from build123d import *

# Parameters (mm, degrees)
F1_DEPTH = 8
F3_DEPTH = 3
F4_R     = 1.5


with BuildPart() as f1:
    # F0 (on Right) → F1 (new body)
    with BuildSketch(Plane.YZ):
        Polygon((0, 14.684157), (-17.555564, 0), (17.444436, 0), align=None)
    extrude(amount=F1_DEPTH)

    # F2 (on face) → F3 (cut)
    with BuildSketch(Plane.YZ.offset(8)):
        Polygon((-0.5, 11.925979), (-12.543837, 1.82), (-7.876665, 1.82), (-4.89646, 4.320689), (-2.798133, 1.82), (-0.5, 3.748363), (-2.598327, 6.249052), (-0.5, 8.009757), align=None)
        Polygon((2.5, 10.174213), (0.5, 11.852412), (0.5, 5.748363), (4.663075, 5.748363), (7.046582, 3.748363), (0.5, 3.748363), (0.5, 1.82), (12.456163, 1.82), (5.391016, 7.748363), (2.5, 7.748363), align=None)
    extrude(amount=-F3_DEPTH, mode=Mode.SUBTRACT)

    # F4
    f4_edges = [f1.edges().sort_by_distance(p)[0] for p in [
        (8, 8.722218, 7.342078),
        (8, -8.777782, 7.342078),
        (8, -0.055564, 0),
    ]]
    fillet(f4_edges, radius=F4_R)


solid = f1.part
The listing builds one solid part. Answer for the finished solid, in the listing's coordinates (mm). A direction names the side the tool comes from. Give positions to 0.01 mm unless a question says otherwise; leave off trailing zeros. Write each loop counter-clockwise with the first axis right and the second up, starting at its lowest first coordinate (ties: lowest second). Pieces come first, ordered by that corner, then holes.
Item 1: Determine the mould class of faces 1 (the flat face through (0, 0, 6)), 2 (the flat face through (6.521, 8.973, 4.743)), 3 (the flat face through (3.204, 8.844, 7.239)), 4 (the cylindrical face through (7.55, -8.63, 6.91)) for opening direction Y: released by +Y, released by -Y, zero draft, split by the parting line, or undercut.
Item 2: Section A-A, the plane x = 6 is taken. Write down the section's boundary in (y, z).
Item 3: Section B-B, the plane x = 1 is taken. Write down the section's boundary in (y, z).
Item 4: Flat-ended cylindrical pins translate along their axes: P1, Ø3.5, axis at x = 7, y = 6, coming from the +Z side; P2, Ø2, axis at x = 7, z = 3, coming from the +Y side; P3, Ø2.5, axis at x = 6.5, y = 2, coming from the +Z side; P4, Ø2, axis at y = 7, z = 12, coming from the -X side. Find the tip coordinate at first contact, or state that the pin passes through.
Item 5: Find the intervals of material crossed by line 1 along Y through (x, z) = (5.75, 2); line 2 along Z through (x, y) = (7.25, 1.5); line 3 along X through (y, z) = (-3.5, 3.5), in increasing order.
Item 6: Which of the six approach directions +Z, -Z, +X, -X, +Y, -Y give full straight-line access (tool end or side, diameter ignored) to faces 5 (the flat face through (3, 0, 0)), 6 (the flat face through (7, -0.5, 10))?
Completed:
1. face 1: zero draft
1. face 2: undercut
1. face 3: released by +Y
1. face 4: released by -Y
2. outline: (-17.56, 0) - (17.44, 0) - (0, 14.68) - close; hole (-12.54, 1.82) - (-7.88, 1.82) - (-4.9, 4.32) - (-2.8, 1.82) - (-0.5, 3.75) - (-2.6, 6.25) - (-0.5, 8.01) - (-0.5, 11.93) - close; hole (0.5, 1.82) - (12.46, 1.82) - (5.39, 7.75) - (2.5, 7.75) - (2.5, 10.17) - (0.5, 11.85) - (0.5, 5.75) - (4.66, 5.75) - (7.05, 3.75) - (0.5, 3.75) - close
3. outline: (-17.56, 0) - (17.44, 0) - (0, 14.68) - close
4. P1: stops at z = 11.07
4. P2: stops at y = 15
4. P3: stops at z = 14.05
4. P4: passes through
5. line 1: y = -15.16 to -12.33, -7.66 to -2.95, -2.58 to 0.5, 12.24 to 15.07
5. line 2: z = 0.2 to 1.82, 3.75 to 5.75, 11.01 to 13.16
5. line 3: x = 0 to 5
6. face 5: -Z, +X, -X, +Y, -Y
6. face 6: +X
